The model under review builds one solid part; all positions refer to its coordinate system, in mm. A direction names the side the tool comes from. Give positions to 0.01 mm unless a question says otherwise; leave off trailing zeros. Order: outer loops, then holes, each group sorted by start corner. A loop starts at its lowest first (then second) coordinate and runs counter-clockwise, first axis right, second up. Notation, with made-up numbers: M -26.75,-15 L 32.25,-15 A18 ccw 32.25,9 Z; hole C 82.25,59 d2. An arc over 180 degrees is marked long. One line per question, with ' | ' between items. Start each with the question number.
1. Wall thickness on L1, parallel to X at y = -5.5, z = 1.65; L2, parallel to Y at x = 12, z = 0.35; L3, parallel to X at y = 24.5, z = 0.4: over which ranges is each line inside the solid? List them lowest first.
2. We need section B-B on x = 13. Write out the cut boundary in (y, z), then the cut area to 3 significant figures.
3. We need section A-A on y = 2. Write out the cut boundary in (x, z), then the cut area to 3 significant figures.
4. Insertion check: P1, Ø0.6, axis at x = -0.5, z = 0, coming from the +Y side; P2, Ø1.2, axis at x = 0, z = 1.5, coming from the +Y side. Each pin has a flat end and moves straight along its axis. Give the tip position at first contact, or say it passes through.
5. The part is to be moulded in two halves that separate along Y. For faces 1 (the face through (43, 29.581, 1)), 2 (the face through (58.087, -11, 1)), 3 (the face through (8.9, -3.6, 0.5)), 4 (the face through (7, -50.419, 1)), say which applies: +Y half, -Y half, draft (parallel to the pull), parting line (faces both ways), or undercut.
6. We need section D-D on y = -18. Write out the cut boundary in (x, z).
7. For faces 5 (the face through (37.59, 10.17, 1.01)), 6 (the face through (28.087, 14, 1)), list the 3-axis set-ups (+Z, -Z, +X, -X, +Y, -Y) from which the entire face can be reached by the end or side of a thin tool; tool diameter is ignored.
8. We need section C-C on z = 1.45. Write out the cut boundary in (x, y).
```python
from build123d import *

# Parameters (mm, degrees)
F0_W     = 100
F0_H     = 80
F1_DEPTH = 2
F2_W     = 40
F2_H     = 31
F3_DEPTH = 2.001
F4_W     = 61
F4_H     = 41
F5_DEPTH = 1.5
F6_R     = 1.524
F6_R_2   = 1.524001
F7_DEPTH = 2.001
F8_W     = 50
F8_H     = 36
F9_DEPTH = 0.501


with BuildPart() as f1:
    # F0 (on Top) → F1 (new body)
    with BuildSketch(Plane.XY):
        with Locations((8.086769, -10.418962)):
            Rectangle(F0_W, F0_H)
    extrude(amount=F1_DEPTH)

    # F2 (on face) → F3 (cut, through all)
    with BuildSketch(Plane.XY.offset(2)):
        with Locations((8.086769, 14.081038)):
            Rectangle(F2_W, F2_H)
    extrude(amount=-F3_DEPTH, mode=Mode.SUBTRACT)

    # F4 (on face) → F5 (cut)
    with BuildSketch(Plane.XY.offset(2)):
        with Locations((9.086769, -21.918962)):
            Rectangle(F4_W, F4_H)
    extrude(amount=-F5_DEPTH, mode=Mode.SUBTRACT)

    # F6 (on face) → F7 (cut, through all)
    with BuildSketch(Plane.XY.offset(2)):
        with Locations((-33.985233, 10.10504)):
            Circle(F6_R)
        with Locations((-22.937232, 10.105039)):
            Circle(F6_R_2)
        with Locations((50.158769, 10.105038)):
            Circle(F6_R)
        with Locations((39.110769, 10.105038)):
            Circle(F6_R)
    extrude(amount=-F7_DEPTH, mode=Mode.SUBTRACT)

    # F8 (on face) → F9 (cut, through all)
    with BuildSketch(Plane.XY.offset(0.5)):
        with Locations((9.086769, -21.918962)):
            Rectangle(F8_W, F8_H)
    extrude(amount=-F9_DEPTH, mode=Mode.SUBTRACT)


solid = f1.part
```
Entries:
1) L1: x = -41.91 to -21.41, 39.59 to 58.09 | L2: y = -50.42 to -39.92, -3.92 to -1.42 | L3: x = -41.91 to -11.91, 28.09 to 58.09
2) outline: M -50.42,0 L -39.92,0 L -39.92,0.5 L -42.42,0.5 L -42.42,2 L -50.42,2 Z; M -3.92,0 L -1.42,0 L -1.42,0.5 L -3.92,0.5 Z | area: 18.5 mm^2
3) outline: M -41.91,0 L -11.91,0 L -11.91,2 L -41.91,2 Z; M 28.09,0 L 58.09,0 L 58.09,2 L 28.09,2 Z | area: 120 mm^2
4) P1: stops at y = -1.42 | P2: stops at y = -42.42
5) face 1: +Y half | face 2: draft | face 3: undercut | face 4: -Y half
6) outline: M -41.91,0 L -15.91,0 L -15.91,0.5 L -21.41,0.5 L -21.41,2 L -41.91,2 Z; M 34.09,0 L 58.09,0 L 58.09,2 L 39.59,2 L 39.59,0.5 L 34.09,0.5 Z
7) face 5: +Z, -Z | face 6: +Z, -Z, +Y
8) outline: M -41.91,-50.42 L 58.09,-50.42 L 58.09,29.58 L 28.09,29.58 L 28.09,-1.42 L 39.59,-1.42 L 39.59,-42.42 L -21.41,-42.42 L -21.41,-1.42 L -11.91,-1.42 L -11.91,29.58 L -41.91,29.58 Z; hole C -33.99,10.11 d3.05; hole C -22.94,10.11 d3.05; hole C 39.11,10.11 d3.05; hole C 50.16,10.11 d3.05
